For this review, use the dimensioned drawing (mm, ordinates from the lowest corner) and the shaded views. A direction names the side the tool comes from. Round coordinates to 2 decimals unless told otherwise and drop trailing zeros. Loops run counter-clockwise (first coordinate to the right, second up) from the corner with the lowest first, then second, coordinate; pieces in that order, holes last. Notation, with made-up numbers: M 0,-37.5 L 12,-37.5 A19 cw 12,-21.5 Z; hole C -11,59 d3. An arc over 180 degrees is marked long. One line per item, written item: value. Start each with the question number.
Item 1: For the marked faces 1 and 2, list the 3-axis set-ups (+Z, -Z, +X, -X, +Y, -Y) from which the entire face can be reached by the end or side of a thin tool; tool diameter is ignored.
Item 2: We need section A-A (y = 4.5). Write out the cut boundary in (x, z), then the cut area to 3 significant figures.
Item 3: We need section D-D (z = 2.75). Write out the cut boundary in (x, y), then the cut area to 3 significant figures.
Item 4: For line 1 along Y through (x, z) = (5, 4.25); line 2 along Y through (x, z) = (3, 4); line 3 along X through (y, z) = (2.25, 7), list the stretches that pass through material, from the lowest coordinate up.
Item 5: Clearance check with flat-ended pins moving along their axes: pin 1 (4 mm diameter, centred on x = 7.5, z = 5, fed in from -Y); pin 2 (3 mm diameter, centred on y = 4, z = 6, fed in from -X); pin 3 (1 mm diameter, centred on x = 6.5, z = 9, fed in from +Y). State where each tip first meets the part, or that it passes through.
Item 6: We need section C-C (z = 9.25). Write out the cut boundary in (x, y), then the cut area to 3 significant figures.
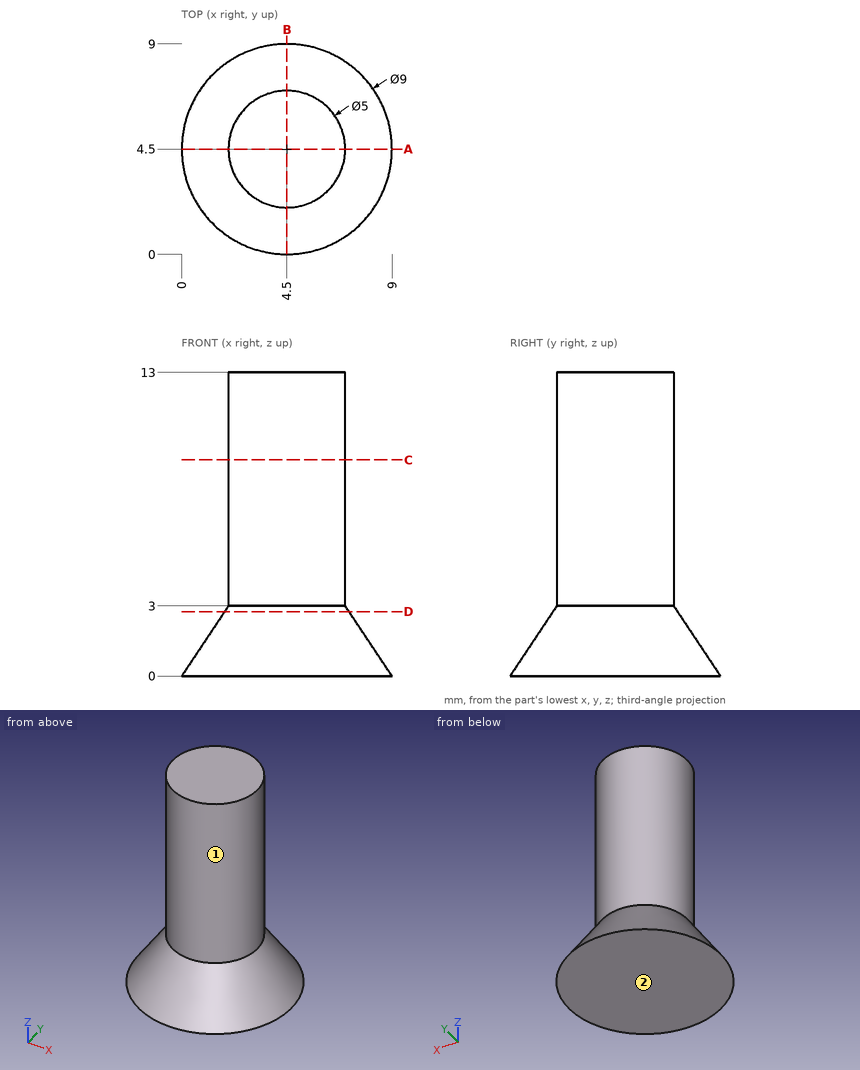
A:
1. face 1: +Z
1. face 2: -Z, +X, -X, +Y, -Y
2. outline: M 0,0 L 9,0 L 7,3 L 7,13 L 2,13 L 2,3 Z
2. area: 71.0 mm2
3. outline: C 4.5,4.5 d5.33
3. area: 22.3 mm2
4. line 1: 2.05 to 6.95
4. line 2: 2.5 to 6.5
4. line 3: 3.41 to 5.59
5. pin 1: y = 2.21
5. pin 2: x = 2
5. pin 3: y = 6.5
6. outline: C 4.5,4.5 d5
6. area: 19.6 mm2
